```python
from build123d import *

# Parameters (mm, degrees)
SKETCH1_W                = 66.22
SKETCH1_H                = 10
SKETCH1_R                = 1.5
BOSS_EXTRUDE1_DEPTH      = 3
BOSS_EXTRUDE2_DEPTH      = 3
BOSS_EXTRUDE2_DEPTH_BACK = 3
SKETCH2_W                = 30
SKETCH2_H                = 30
SKETCH3_R                = 1.5
CUT_EXTRUDE1_DEPTH       = 72.76188682


with BuildPart() as part:
    # Sketch1 → Boss-Extrude1 (new body)
    with BuildSketch(Plane.XY):
        with Locations((30.11, 5)):
            Rectangle(SKETCH1_W, SKETCH1_H)
        with Locations((0, 5)):
            Circle(SKETCH1_R, mode=Mode.SUBTRACT)
        with Locations((60.22, 5)):
            Circle(SKETCH1_R, mode=Mode.SUBTRACT)
    extrude(amount=BOSS_EXTRUDE1_DEPTH)

    # Sketch2 → Boss-Extrude2 (add, two sides: drawn at the far end of the back side and taken through both)
    with BuildSketch(Plane(origin=(0, 5, 0), x_dir=(1, 0, 0), z_dir=(0, 1, 0)).offset(-BOSS_EXTRUDE2_DEPTH_BACK)):
        with Locations((30.22, -18)):
            Rectangle(SKETCH2_W, SKETCH2_H)
    extrude(amount=BOSS_EXTRUDE2_DEPTH + BOSS_EXTRUDE2_DEPTH_BACK)

    # Sketch3 → Cut-Extrude1 (cut, through all)
    with BuildSketch(Plane.XZ.offset(-2)):
        with Locations(Location((19.72, 30, 0), (0, 0, 270))):
            Circle(SKETCH3_R)
        with Locations(Location((40.53, 30, 0), (0, 0, 270))):
            Circle(SKETCH3_R)
    extrude(amount=-CUT_EXTRUDE1_DEPTH, mode=Mode.SUBTRACT)


solid = part.part
```
Source: CAD feature listing. Evaluate the final solid. Frame: model axes, mm. A direction names the side the tool comes from. Coordinates: 2 decimals unless noted, no trailing zeros. Loops run counter-clockwise (first coordinate to the right, second up) from the corner with the lowest first, then second, coordinate; pieces in that order, holes last. Notation, with made-up numbers: (-16.75, 21.25) - (22.25, 21.25) arc R25 ccw to (22.25, 55.25) - close; hole circle Ø11 at (49, -32). An arc over 180 degrees is marked (long way). Answer as CSV lines item,"result".
1. Section D-D (z = 7). Return loops of the section in (x, y).
Established:
outline,"(15.22, 2) - (45.22, 2) - (45.22, 8) - (15.22, 8) - close"
2. Mould query, pull axis X, two halves, no side actions, for faces 1 (the cylindrical face through (58.72, 5.07, 1.48)), 2 (the flat face through (29.6, 8.4, 3)), 3 (the flat face through (15.22, 5, 18)). Classes: released by +X, released by -X, zero draft, split by the parting line, or undercut.
Established:
face 1,"undercut"
face 2,"zero draft"
face 3,"released by -X"
3. Contact query for flat-ended pins moving along their axis: pin 1 (3 mm diameter, centred on x = 50, z = 5.5, fed in from -Y); pin 2 (5 mm diameter, centred on x = 19.72, z = 30, fed in from +Y); pin 3 (15 mm diameter, centred on x = 32.5, z = 16, fed in from -Y); pin 4 (5 mm diameter, centred on y = 4, z = 11, fed in from +X). Output: stop coordinate, or through.
Established:
pin 1,"passes through"
pin 2,"stops at y = 8"
pin 3,"stops at y = 2"
pin 4,"stops at x = 45.22"
4. Section A-A (z = 30). Return loops of the section in (x, y).
Established:
outline,"(15.22, 2) - (18.22, 2) - (18.22, 8) - (15.22, 8) - close; (21.22, 2) - (39.03, 2) - (39.03, 8) - (21.22, 8) - close; (42.03, 2) - (45.22, 2) - (45.22, 8) - (42.03, 8) - close"
5. Section C-C (x = 60.22). Return loops of the section in (y, z).
Established:
outline,"(0, 0) - (3.5, 0) - (3.5, 3) - (0, 3) - close; (6.5, 0) - (10, 0) - (10, 3) - (6.5, 3) - close"
6. Reachability of faces 4 (the flat face through (30, 8, 18)), 5 (the flat face through (30, 2, 18)), 6 (the flat face through (30, 10, 1)), 7 (the flat face through (30, 5, 0)), 8 (the flat face through (45.22, 5, 18)) from +Z, -Z, +X, -X, +Y, -Y: full face, straight path, thin tool, end or side. Return the list, or none.
Established:
face 4,"+Z, +X, -X, +Y"
face 5,"+Z, +X, -X, -Y"
face 6,"+Z, -Z, +X, -X, +Y"
face 7,"-Z, +X, -X, +Y, -Y"
face 8,"+Z, +X, +Y, -Y"
7. Ray query, line 1 (Y direction, x = 0, z = 1.85); line 2 (X direction, y = 3.9, z = 30); line 3 (X direction, y = 5, z = 13). Return the intervals inside material, ascending.
Established:
line 1,"y = 0 to 3.5, 6.5 to 10"
line 2,"x = 15.22 to 18.22, 21.22 to 39.03, 42.03 to 45.22"
line 3,"x = 15.22 to 45.22"
8. Section B-B (x = 40.53). Return loops of the section in (y, z), then the cut area to 3 significant figures.
Established:
outline,"(0, 0) - (10, 0) - (10, 3) - (8, 3) - (8, 28.5) - (2, 28.5) - (2, 3) - (0, 3) - close; (2, 31.5) - (8, 31.5) - (8, 33) - (2, 33) - close"
area,"192 mm2"
